Could you check a few things on this model? Use its own coordinates, in mm. Face numbers are marked on the shaded views. A direction names the side the tool comes from. Give positions to 0.01 mm unless a question says otherwise; leave off trailing zeros. Order: outer loops, then holes, each group sorted by start corner. A loop starts at its lowest first (then second) coordinate and runs counter-clockwise, first axis right, second up. Notation, with made-up numbers: (87, -29) -> (107, -29) arc R15 ccw to (107, -16) -> close; hole circle Ø3 at (17, -28.5). An arc over 180 degrees is marked (long way). Write each question's results on one line, items separated by ' | '.
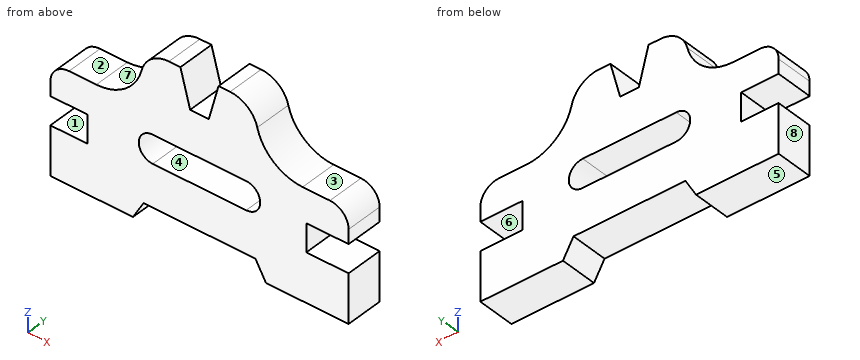
```python
from build123d import *

# Parameters (mm, degrees)
F1_DEPTH = 25.4
F3_DEPTH = 25.4


with BuildPart() as f1:
    # F0 (on Front) → F1 (new body)
    with BuildSketch(Plane.XZ):
        with BuildLine():
            Line((60.532423, 0), (60.532423, 19.05))
            Line((60.532423, 19.05), (89.266929, 19.05))
            Line((89.266929, 19.05), (89.266929, 28.702))
            ThreePointArc((89.266929, 28.702), (85.547185, 37.682256), (76.566929, 41.402))
            Line((76.566929, 41.402), (58.024929, 41.402))
            ThreePointArc((58.024929, 41.402), (38.452915, 48.152025), (27.20289, 65.532))
            ThreePointArc((27.20289, 65.532), (20.452875, 75.959985), (8.709666, 80.01))
            Line((8.709666, 80.01), (0.872661, 80.01))
            Line((0.872661, 80.01), (-5.729071, 55.372))
            Line((-5.729071, 55.372), (-18.429071, 55.372))
            Line((-18.429071, 55.372), (-25.030803, 80.01))
            Line((-25.030803, 80.01), (-32.867808, 80.01))
            ThreePointArc((-32.867808, 80.01), (-44.611017, 75.959985), (-51.361032, 65.532))
            ThreePointArc((-51.361032, 65.532), (-62.611057, 48.152025), (-82.183071, 41.402))
            Line((-82.183071, 41.402), (-100.725071, 41.402))
            ThreePointArc((-100.725071, 41.402), (-109.705327, 37.682256), (-113.425071, 28.702))
            Line((-113.425071, 28.702), (-113.425071, 19.05))
            Line((-113.425071, 19.05), (-88.025071, 19.05))
            Line((-88.025071, 19.05), (-88.025071, 0))
            Line((-88.025071, 0), (-113.425071, 0))
            Line((-113.425071, 0), (-113.425071, -33.02))
            Line((-113.425071, -33.02), (-57.291071, -33.02))
            Line((-57.291071, -33.02), (-50.10537, -20.574))
            Line((-50.10537, -20.574), (25.947228, -20.574))
            Line((25.947228, -20.574), (33.132929, -33.02))
            Line((33.132929, -33.02), (89.266929, -33.02))
            Line((89.266929, -33.02), (89.266929, 0))
            Line((89.266929, 0), (60.532423, 0))
        make_face()
    extrude(amount=F1_DEPTH)

    # F2 (on face) + F0 (on Front) → F3 (cut)
    with BuildSketch(Plane.XZ.offset(25.4)):
        with BuildLine():
            Line((19.670929, 27.051), (-43.829071, 27.051))
            ThreePointArc((-43.829071, 27.051), (-53.354071, 17.526), (-43.829071, 8.001))
            Line((-43.829071, 8.001), (19.670929, 8.001))
            ThreePointArc((19.670929, 8.001), (29.195929, 17.526), (19.670929, 27.051))
        make_face()
    with BuildSketch(Plane.XZ):
        with BuildLine():
            Line((60.532423, 0), (60.532423, 19.05))
            Line((60.532423, 19.05), (89.266929, 19.05))
            Line((89.266929, 19.05), (89.266929, 28.702))
            ThreePointArc((89.266929, 28.702), (85.547185, 37.682256), (76.566929, 41.402))
            Line((76.566929, 41.402), (58.024929, 41.402))
            ThreePointArc((58.024929, 41.402), (38.452915, 48.152025), (27.20289, 65.532))
            ThreePointArc((27.20289, 65.532), (20.452875, 75.959985), (8.709666, 80.01))
            Line((8.709666, 80.01), (0.872661, 80.01))
            Line((0.872661, 80.01), (-5.729071, 55.372))
            Line((-5.729071, 55.372), (-18.429071, 55.372))
            Line((-18.429071, 55.372), (-25.030803, 80.01))
            Line((-25.030803, 80.01), (-32.867808, 80.01))
            ThreePointArc((-32.867808, 80.01), (-44.611017, 75.959985), (-51.361032, 65.532))
            ThreePointArc((-51.361032, 65.532), (-62.611057, 48.152025), (-82.183071, 41.402))
            Line((-82.183071, 41.402), (-100.725071, 41.402))
            ThreePointArc((-100.725071, 41.402), (-109.705327, 37.682256), (-113.425071, 28.702))
            Line((-113.425071, 28.702), (-113.425071, 19.05))
            Line((-113.425071, 19.05), (-88.025071, 19.05))
            Line((-88.025071, 19.05), (-88.025071, 0))
            Line((-88.025071, 0), (-113.425071, 0))
            Line((-113.425071, 0), (-113.425071, -33.02))
            Line((-113.425071, -33.02), (-57.291071, -33.02))
            Line((-57.291071, -33.02), (-50.10537, -20.574))
            Line((-50.10537, -20.574), (25.947228, -20.574))
            Line((25.947228, -20.574), (33.132929, -33.02))
            Line((33.132929, -33.02), (89.266929, -33.02))
            Line((89.266929, -33.02), (89.266929, 0))
            Line((89.266929, 0), (60.532423, 0))
        make_face()
    extrude(amount=-F3_DEPTH, mode=Mode.SUBTRACT)


solid = f1.part
```
Q1. I need wall thicknesses on line 1 along Z through (x, y) = (6.5, -9.5); line 2 along Z through (x, y) = (74.5, -19.5); line 3 along X through (y, z) = (-16.25, 18). Which ranges of each line are inside material? Lowest first, please.
Here are the results:
line 1: z = -20.57 to 8, 27.05 to 80.01 | line 2: z = -33.02 to 0, 19.05 to 41.4 | line 3: x = -88.03 to -53.34, 29.18 to 60.53
Q2. Suppose I cut it at D-D on z = 38. Please give me the cut outline in (x, y), and give its area (3 significant figures).
Here are the results:
outline: (-109.38, -25.4) -> (85.22, -25.4) -> (85.22, 0) -> (-109.38, 0) -> close | area: 4,940 mm²
Q3. Suppose I cut it at A-A on x = 66.5. Please give me the cut outline in (y, z).
Here are the results:
outline: (-25.4, -33.02) -> (0, -33.02) -> (0, 0) -> (-25.4, 0) -> close; (-25.4, 19.05) -> (0, 19.05) -> (0, 41.4) -> (-25.4, 41.4) -> close
Q4. Thinking about a two-plate mould opening in Z: for the marked faces 5, 6, 7 and 8, which applies, +Z half, -Z half, draft (parallel to the pull), parting line (faces both ways), or undercut?
Here are the results:
face 5: -Z half | face 6: undercut | face 7: +Z half | face 8: draft
Q5. Suppose I cut it at C-C on z = -25. Please give me the cut outline in (x, y), and give its area (3 significant figures).
Here are the results:
outline: (-113.43, -25.4) -> (-52.66, -25.4) -> (-52.66, 0) -> (-113.43, 0) -> close; (28.5, -25.4) -> (89.27, -25.4) -> (89.27, 0) -> (28.5, 0) -> close | area: 3,090 mm²
Q6. For the marked faces 1, 2, 3 and 4, which set-ups out of +Z, -Z, +X, -X, +Y, -Y let a thin tool reach every point of the face, with its end or its side?
Here are the results:
face 1: -X, +Y, -Y | face 2: +Z, -X, +Y, -Y | face 3: +Z, +X, +Y, -Y | face 4: +Y, -Y
Q7. I'm going to push flat-ended pins straight in: pin 1 Ø2 at (x, z) = (-6.5, 60.5) entering from -Y; pin 2 Ø2 at (y, z) = (-12.5, 9) entering from +X; pin 3 Ø6 at (y, z) = (-15.5, 14) entering from -X; pin 4 Ø2 at (x, y) = (-40, -17) entering from -Z. Where does each tip first touch, or does it pass through?
Here are the results:
pin 1: passes through | pin 2: stops at x = 60.53 | pin 3: stops at x = -88.03 | pin 4: stops at z = -20.57
